Read the model definition and answer for the solid it produces. Units are mm, in the model's axes. Face numbers are marked on the shaded views. A direction names the side the tool comes from. Coordinates: 2 decimals unless noted, no trailing zeros. Write each loop counter-clockwise with the first axis right and the second up, starting at its lowest first coordinate (ties: lowest second). Pieces come first, ordered by that corner, then holes. Notation, with made-up numbers: (-39, 46.5) -> (-15, 46.5) arc R23 ccw to (-15, 72.5) -> close; hole circle Ø2 at (-25.5, -31.5). An arc over 180 degrees is marked (long way). One line per item, written item: value. Start each with the question number.
1. Given P1, Ø4, axis at x = -27.5, y = 26.5, coming from the -Z side; P2, Ø2.5, axis at x = 26.5, y = 26, coming from the -Z side; P3, Ø17.5, axis at x = 0, y = 0, coming from the +Z side; P4, Ø3, axis at x = 4, z = -30, coming from the +Y side, each flat-ended and moving along its own axis, determine where each tip first touches the part or whether it passes through.
2. Consider line 1 along Y through (x, z) = (-7, -4.5); line 2 along Y through (x, z) = (34, 2). Determine where each line is inside the solid, lowest interval first.
3. For the marked faces 1, 2 and 3, determine the directions among +Z, -Z, +X, -X, +Y, -Y from which every point of the face is accessible in a straight line to the end or side of a thin tool.
4. Find section D-D, the plane x = -13. Write down the section's boundary in (y, z).
5. Find section C-C, the plane z = -31. Write down the section's boundary in (x, y).
6. For a pull along Y with two mould halves and no side action, classify the marked faces 4, 5 and 6 as pulls with the +Y half, pulls with the -Y half, needs draft (parallel to the pull), parting line crosses it, or undercut.
7. Find section B-B, the plane z = 1.5. Write down the section's boundary in (x, y).
8. Find section A-A, the plane y = -34. Write down the section's boundary in (x, z), and give its area (3 significant figures).
```python
from build123d import *

# Parameters (mm, degrees)
SKETCH_W                   = 74
SKETCH_H                   = 74
PAD_DEPTH                  = 5
SKETCH002_W                = 64
SKETCH002_H                = 64
SKETCH002_W_2              = 60
SKETCH002_H_2              = 60
PAD001_DEPTH               = 40
SKETCH003_R                = 1.5
POCKET_DEPTH               = 232.834272
PAD002_DEPTH               = 37
SKETCH005_R                = 2.4
POCKET001_DEPTH            = 10
SKETCH003_MIRRORED_2_R     = 1.5
POCKET_MIRRORED_2_DEPTH    = 232.834272
PAD002_MIRRORED_2_DEPTH    = 37
SKETCH005_MIRRORED_2_R     = 2.4
POCKET001_MIRRORED_2_DEPTH = 10
SKETCH006_R                = 14.5
SKETCH006_R_2              = 2.5
POCKET002_DEPTH            = 45.001
SKETCH007_W                = 2.5
SKETCH007_H                = 5
PAD003_DEPTH               = 8


with BuildPart() as part:
    # Sketch → Pad (new body)
    with BuildSketch(Plane.XY):
        Rectangle(SKETCH_W, SKETCH_H)
    extrude(amount=PAD_DEPTH)

    # Sketch002 (on Face5 of Pad) → Pad001 (join)
    with BuildSketch(Plane(origin=(0, 0, 0), x_dir=(1, 0, 0), z_dir=(0, 0, -1))):
        Rectangle(SKETCH002_W, SKETCH002_H)
        Rectangle(SKETCH002_W_2, SKETCH002_H_2, mode=Mode.SUBTRACT)
    extrude(amount=PAD001_DEPTH)

    # Sketch003 (on Face4 of Pad001) → Pocket (cut, through all)
    with BuildSketch(Plane(origin=(0, 0, 0), x_dir=(1, 0, 0), z_dir=(0, 0, -1))):
        with Locations((-34, 34)):
            Circle(SKETCH003_R)
    pocket = extrude(amount=-POCKET_DEPTH, mode=Mode.SUBTRACT)

    # Sketch004 (on Face17 of Pocket) → Pad002 (join)
    with BuildSketch(Plane(origin=(0, 0, 0), x_dir=(1, 0, 0), z_dir=(0, 0, -1))):
        with BuildLine():
            ThreePointArc((-30, 22), (-24.343146, 24.343146), (-22, 30))
            Line((-30, 30), (-22, 30))
            Line((-30, 30), (-30, 22))
        make_face()
    pad002 = extrude(amount=PAD002_DEPTH)

    # Sketch005 (on Face17 of Pad002) → Pocket001 (cut)
    with BuildSketch(Plane(origin=(0, 0, -37), x_dir=(1, 0, 0), z_dir=(0, 0, -1))):
        with Locations((-27, 27)):
            Circle(SKETCH005_R)
    pocket001 = extrude(amount=-POCKET001_DEPTH, mode=Mode.SUBTRACT)

    # Sketch003 Mirrored 2 → Pocket Mirrored 2 (cut, through all)
    with BuildSketch(Plane(origin=(0, 0, 0), x_dir=(-1, 0, 0), z_dir=(0, 0, 1))):
        with Locations((-34, 34)):
            Circle(SKETCH003_MIRRORED_2_R)
    pocket_mirrored_2 = extrude(amount=POCKET_MIRRORED_2_DEPTH, mode=Mode.SUBTRACT)

    # Sketch004 Mirrored 2 → Pad002 Mirrored 2 (add)
    with BuildSketch(Plane(origin=(0, 0, 0), x_dir=(-1, 0, 0), z_dir=(0, 0, 1))):
        with BuildLine():
            ThreePointArc((-30, 22), (-24.343146, 24.343146), (-22, 30))
            Line((-30, 30), (-22, 30))
            Line((-30, 30), (-30, 22))
        make_face()
    pad002_mirrored_2 = extrude(amount=-PAD002_MIRRORED_2_DEPTH)

    # Sketch005 Mirrored 2 → Pocket001 Mirrored 2 (cut)
    with BuildSketch(Plane(origin=(0, 0, -37), x_dir=(-1, 0, 0), z_dir=(0, 0, 1))):
        with Locations((-27, 27)):
            Circle(SKETCH005_MIRRORED_2_R)
    pocket001_mirrored_2 = extrude(amount=POCKET001_MIRRORED_2_DEPTH, mode=Mode.SUBTRACT)

    # Mirrored001: Pocket, Pad002, Pocket001, Pocket Mirrored 2, Pad002 Mirrored 2, Pocket001 Mirrored 2 across Sketch003 H_Axis
    add(pocket.mirror(Plane(origin=(0, 0, 0), x_dir=(0, 0, -1), z_dir=(0, -1, 0))), mode=Mode.SUBTRACT)
    add(pad002.mirror(Plane(origin=(0, 0, 0), x_dir=(0, 0, -1), z_dir=(0, -1, 0))))
    add(pocket001.mirror(Plane(origin=(0, 0, 0), x_dir=(0, 0, -1), z_dir=(0, -1, 0))), mode=Mode.SUBTRACT)
    add(pocket_mirrored_2.mirror(Plane(origin=(0, 0, 0), x_dir=(0, 0, -1), z_dir=(0, -1, 0))), mode=Mode.SUBTRACT)
    add(pad002_mirrored_2.mirror(Plane(origin=(0, 0, 0), x_dir=(0, 0, -1), z_dir=(0, -1, 0))))
    add(pocket001_mirrored_2.mirror(Plane(origin=(0, 0, 0), x_dir=(0, 0, -1), z_dir=(0, -1, 0))), mode=Mode.SUBTRACT)

    # Sketch006 (on Face36 of MultiTransform) → Pocket002 (cut, through all)
    with BuildSketch(Plane.XY.offset(5)):
        Circle(SKETCH006_R)
        with Locations((0, 22)):
            Circle(SKETCH006_R_2)
    extrude(amount=-POCKET002_DEPTH, mode=Mode.SUBTRACT)

    # Sketch007 (on Face4 of Pocket002) → Pad003 (join)
    with BuildSketch(Plane(origin=(0, 0, 0), x_dir=(1, 0, 0), z_dir=(0, 0, -1))):
        with Locations((-7.25, -22)):
            Rectangle(SKETCH007_W, SKETCH007_H)
    extrude(amount=PAD003_DEPTH)


solid = part.part
```
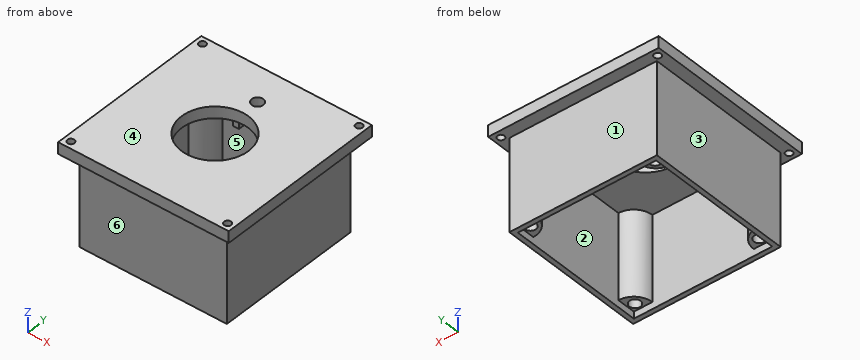
Answer block:
1. P1: stops at z = -37
1. P2: stops at z = -27
1. P3: passes through
1. P4: stops at y = 32
2. line 1: y = -32 to -30, 19.5 to 24.5, 30 to 32
2. line 2: y = -37 to -35.5, -32.5 to 32.5, 35.5 to 37
3. face 1: -Z, +X, -X, +Y
3. face 2: -Z
3. face 3: -Z, -X, +Y, -Y
4. outline: (-37, 0) -> (-32, 0) -> (-32, -40) -> (-30, -40) -> (-30, 0) -> (-6.42, 0) -> (-6.42, 5) -> (-37, 5) -> close; (6.42, 0) -> (30, 0) -> (30, -40) -> (32, -40) -> (32, 0) -> (37, 0) -> (37, 5) -> (6.42, 5) -> close
5. outline: (-32, -32) -> (32, -32) -> (32, 32) -> (-32, 32) -> close; hole (-30, -22) arc R8 cw to (-22, -30) -> (22, -30) arc R8 cw to (30, -22) -> (30, 22) arc R8 cw to (22, 30) -> (-22, 30) arc R8 cw to (-30, 22) -> close; hole circle Ø4.8 at (-27, -27); hole circle Ø4.8 at (-27, 27); hole circle Ø4.8 at (27, -27); hole circle Ø4.8 at (27, 27)
6. face 4: needs draft
6. face 5: undercut
6. face 6: pulls with the -Y half
7. outline: (-37, -37) -> (37, -37) -> (37, 37) -> (-37, 37) -> close; hole circle Ø3 at (-34, -34); hole circle Ø3 at (-34, 34); hole circle Ø29 at (0, 0); hole circle Ø5 at (0, 22); hole circle Ø3 at (34, -34); hole circle Ø3 at (34, 34)
8. outline: (-37, 0) -> (-35.5, 0) -> (-35.5, 5) -> (-37, 5) -> close; (-32.5, 0) -> (32.5, 0) -> (32.5, 5) -> (-32.5, 5) -> close; (35.5, 0) -> (37, 0) -> (37, 5) -> (35.5, 5) -> close
8. area: 340 mm2
